Verification items for the finished model (mm, model axes). A direction names the side the tool comes from. Round coordinates to 2 decimals unless told otherwise and drop trailing zeros. Order: outer loops, then holes, each group sorted by start corner. A loop starts at its lowest first (then second) coordinate and runs counter-clockwise, first axis right, second up. Notation, with made-up numbers: (63, 2.5) -> (78, 2.5) arc R16 cw to (78, 9.5) -> close; hole circle Ø11 at (25, -12). An arc over 180 degrees is marked (long way). Put each result on its own line as item: value.
from build123d import *

# Parameters (mm, degrees)
CROQUIS1_R              = 24.9
CROQUIS1_R_2            = 2.4
SALIENTE_EXTRUIR1_DEPTH = 8.5
CROQUIS2_R              = 4.25
SALIENTE_EXTRUIR2_DEPTH = 15
CHAFL_N1_SIZE           = 1


with BuildPart() as part:
    # Croquis1 → Saliente-Extruir1 (new body)
    with BuildSketch(Plane(origin=(0, 0, 0), x_dir=(0, 0, -1), z_dir=(1, 0, 0))):
        Circle(CROQUIS1_R)
        Circle(CROQUIS1_R_2, mode=Mode.SUBTRACT)
    extrude(amount=SALIENTE_EXTRUIR1_DEPTH)

    # Croquis2 → Saliente-Extruir2 (add)
    with BuildSketch(Plane(origin=(8.5, 0, 0), x_dir=(0, 0, -1), z_dir=(1, 0, 0))):
        with Locations((-15.09387296, 10.696962141)):
            Circle(CROQUIS2_R)
    extrude(amount=SALIENTE_EXTRUIR2_DEPTH)

    # Chaflán1
    chafl_n1_edges = [part.edges().sort_by_distance(p)[0] for p in [
        (8.5, 10.696962141, 19.34387296),
    ]]
    chamfer(chafl_n1_edges, length=CHAFL_N1_SIZE)


solid = part.part
Item 1: Section check A-A on y = 0. Record the boundary of the cut face in (x, z), then the cut area to 4 significant figures.
Check sheet entries:
outline: (0, -24.9) -> (8.5, -24.9) -> (8.5, -2.4) -> (0, -2.4) -> close; (0, 2.4) -> (8.5, 2.4) -> (8.5, 24.9) -> (0, 24.9) -> close
area: 382.5 mm^2
Item 2: Gauge pin test, flat ends, axial feed: pin 1 Ø4 at (y, z) = (17.5, -18.5) entering from +X; pin 2 Ø3 at (x, y) = (8, -12.5) entering from +Z; pin 3 Ø12 at (x, z) = (3, 18) entering from +Y. Record the tip position at first contact, or that the pin passes through.
Check sheet entries:
pin 1: stops at x = 8.5
pin 2: stops at z = 22.34
pin 3: stops at y = 21.82
Item 3: Section check C-C on x = 3.5. Record the boundary of the cut face in (y, z).
Check sheet entries:
outline: circle Ø49.8 at (0, 0); hole circle Ø4.8 at (0, 0)
Item 4: Tool access check on faces 4 (the cylindrical face through (16.4, 11.97, 11.04)), 5 (the flat face through (23.5, 11, 15)). Record the directions out of +Z, -Z, +X, -X, +Y, -Y that give a thin tool (end or side, any length) a straight path to the whole face; none if there is none.
Check sheet entries:
face 4: +X
face 5: +Z, -Z, +X, +Y, -Y
Item 5: Section check D-D on y = 21. Record the boundary of the cut face in (x, z).
Check sheet entries:
outline: (0, -13.38) -> (8.5, -13.38) -> (8.5, 13.38) -> (0, 13.38) -> close
Item 6: Material ranges on L1, parallel to Y at x = 3.5, z = 0; L2, parallel to X at y = 1, z = -23; L3, parallel to Z at x = 12.25, y = 10.5, recorded low to high. Write a range as [from, to].
Check sheet entries:
L1: y = [-24.9, -2.4], [2.4, 24.9]
L2: x = [0, 8.5]
L3: z = [10.85, 19.34]
Item 7: Release check for a two-part mould opening along Z. For faces 1 (the cylindrical face through (4.19, 16.83, 18.35)), 2 (the cylindrical face through (4.19, 2.024, -1.29)), 3 (the flat face through (0, 0, -5)) record: +Z half, -Z half, draft (parallel to the pull), parting line (faces both ways), or undercut.
Check sheet entries:
face 1: parting line
face 2: undercut
face 3: draft
